Model file for the job. Use its own axes, mm. Face numbers are marked on the shaded views. A direction names the side the tool comes from. Round coordinates to 2 decimals unless told otherwise and drop trailing zeros. Order: outer loops, then holes, each group sorted by start corner. A loop starts at its lowest first (then second) coordinate and runs counter-clockwise, first axis right, second up. Notation, with made-up numbers: M 33.25,33 L 84.25,33 A20 cw 84.25,64 Z; hole C 32.5,36 d6. An arc over 180 degrees is marked long. Return JSON: item names as keys, results as strings. Group by question number.
Item 1: Slice it at A-A on x = 0. Write the cut outline in (y, z), then the cut area to 3 significant figures.
Item 2: Which spindle directions (+Z, -Z, +X, -X, +Y, -Y) get a long thin tool onto all of the face, cutting with end or side? Do the marked faces 4 and 5. Say none if no direction does.
Item 3: Slice it at D-D on x = -8.25. Write the cut outline in (y, z), then the cut area to 3 significant figures.
Item 4: Probe line 1 along X through (y, z) = (0.5, 0.25); line 2 along Z through (x, y) = (-6.75, -0.45); line 3 along X through (y, z) = (0.75, -7). List the from-to ranges inside material, lowest first.
Item 5: Slice it at C-C on y = -1. Write the cut outline in (x, z).
Item 6: Slice it at B-B on z = 0. Write the cut outline in (x, y), then the cut area to 3 significant figures.
Item 7: Pull direction Z, two halves, no side cores. Call the marked faces 1, 2 and 3: pulls with the +Z half, pulls with the -Z half, needs draft (parallel to the pull), parting line crosses it, or undercut.
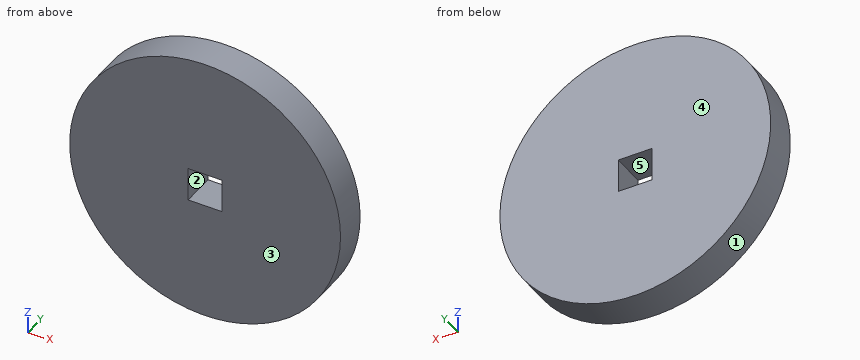
from build123d import *

# Parameters (mm, degrees)
F0_R     = 12.7
F1_DEPTH = 1.5875
F2_W     = 3.175
F2_H     = 3.175
F3_DEPTH = 3.176


with BuildPart() as f1:
    # F0 (on Front) → F1 (new body, symmetric)
    with BuildSketch(Plane.XZ):
        Circle(F0_R)
    extrude(amount=F1_DEPTH, both=True)

    # F2 (on face) → F3 (cut, through all)
    with BuildSketch(Plane(origin=(0, 1.5875, 0), x_dir=(-1, 0, 0), z_dir=(0, 1, 0))):
        Rectangle(F2_W, F2_H)
    extrude(amount=-F3_DEPTH, mode=Mode.SUBTRACT)


solid = f1.part
Output values:
{
 "1": {"outline": "M -1.59,-12.7 L 1.59,-12.7 L 1.59,-1.59 L -1.59,-1.59 Z; M -1.59,1.59 L 1.59,1.59 L 1.59,12.7 L -1.59,12.7 Z", "area": "70.6 mm²"},
 "2": {"face 4": "+Z, -Z, +X, -X, +Y", "face 5": "+Y, -Y"},
 "3": {"outline": "M -1.59,-9.66 L 1.59,-9.66 L 1.59,9.66 L -1.59,9.66 Z", "area": "61.3 mm²"},
 "4": {"line 1": "-12.7 to -1.59, 1.59 to 12.7", "line 2": "-10.76 to 10.76", "line 3": "-10.6 to 10.6"},
 "5": {"outline": "C 0,0 d25.4; hole M -1.59,-1.59 L 1.59,-1.59 L 1.59,1.59 L -1.59,1.59 Z"},
 "6": {"outline": "M -12.7,-1.59 L -1.59,-1.59 L -1.59,1.59 L -12.7,1.59 Z; M 1.59,-1.59 L 12.7,-1.59 L 12.7,1.59 L 1.59,1.59 Z", "area": "70.6 mm²"},
 "7": {"face 1": "parting line crosses it", "face 2": "undercut", "face 3": "needs draft"}
}
